Design review of the part built by this model. Coordinates are the model's own, in mm. Coordinates: 2 decimals unless noted, no trailing zeros. Write each loop counter-clockwise with the first axis right and the second up, starting at its lowest first coordinate (ties: lowest second). Pieces come first, ordered by that corner, then holes.
Q1. Take a section at A-A, the plane z = 852. Write out the cut boundary in (x, y).
Q2. For L1, parallel to X at y = -0.75, z = 315; L2, parallel to X at y = -3.5, z = 387.5, list the stretches that pass through material, from the lowest coordinate up.
Q3. Take a section at B-B, the plane x = -172.5. Write out the cut boundary in (y, z), plus the area to 3 significant figures.
Q4. For pin 1 Ø1.5 at (y, z) = (-13.5, 556) entering from +X; pin 2 Ø6 at (x, z) = (-119.6, 1082.72) entering from -Y; pin 3 Ø2 at (y, z) = (-11.5, 279) entering from +X, all flat-tipped, find the tip position at first contact; note any pin that passes through.
from build123d import *

# Parameters (mm, degrees)
F2_DEPTH = 18.288
F4_D     = 10
F4_DEPTH = 11.5
F4_TIP   = 3.0043030951


# Not quite as in the source:
# - a variable given as a bare number and used for a length is read in inches; the dataset says mm whatever the document's units were


with BuildPart() as f2:
    # F0 (on Front) → F2 (new body)
    with BuildSketch(Plane.XZ):
        Polygon((-304.6112403404, 1131.9026269978), (-304.6112403404, -87.2973730022), (-228.4112403404, -87.2973730022), (-101.4112403404, 1131.9026269978), align=None)
    extrude(amount=F2_DEPTH)

    # F4
    with Locations(Plane.XZ.offset(18.288)):
        with Locations((-119.6044687363, 1082.7228909215), (-122.9198634326, 1050.895101837)):
            Hole(F4_D / 2, depth=F4_DEPTH)
            with Locations((0, 0, -(F4_DEPTH + F4_TIP / 2))):  # 118° drill point
                Cone(0, F4_D / 2, F4_TIP, mode=Mode.SUBTRACT)


solid = f2.part
Responses:
1. outline: (-304.61, -18.29) - (-130.57, -18.29) - (-130.57, 0) - (-304.61, 0) - close
2. L1: x = -304.61 to -186.51
2. L2: x = -304.61 to -178.95
3. outline: (-18.29, 449.45) - (0, 449.45) - (0, 1131.9) - (-18.29, 1131.9) - close
3. area: 12,500 mm2
4. pin 1: stops at x = -161.32
4. pin 2: stops at y = -5.59
4. pin 3: stops at x = -190.15
